Geometry check sheet. Reference: the model listing, model coordinates, mm. A direction names the side the tool comes from. Round coordinates to 2 decimals unless told otherwise and drop trailing zeros. Order: outer loops, then holes, each group sorted by start corner. A loop starts at its lowest first (then second) coordinate and runs counter-clockwise, first axis right, second up.
(1) Gauge pin test, flat ends, axial feed: P1, Ø3, axis at x = 28, y = -54, coming from the -Z side; P2, Ø8, axis at y = -20.5, z = 7.5, coming from the +X side; P3, Ø3, axis at y = -16.5, z = 34.5, coming from the +X side. Record the tip position at first contact, or that the pin passes through.
(2) Cross-section at C-C on x = 9.5. Enter the section's corners in (y, z).
(3) Cross-section at A-A on z = 12.7. Enter the section's corners in (x, y) (3 decimals), and give its area (3 significant figures).
(4) Cross-section at B-B on y = -12.7. Enter the section's corners in (x, z) (3 decimals), and give its area (3 significant figures).
(5) Thickness scan on L1, parallel to Z at x = 2.5, y = -76.2 (3 decimals); L2, parallel to Y at x = 5, z = 15.5; L3, parallel to Z at x = 36, y = -14. Record the ranges inside material, lowest first.
(6) Set-up check for faces 5 (the face through (11.81, -80.9, 35.67)), 6 (the face through (34, -44, 32.539)): record each of +Z, -Z, +X, -X, +Y, -Y from which the full face is reachable in a straight line by a thin tool's end or side.
(7) Cross-section at D-D on y = -56. Enter the section's corners in (x, z).
(8) Draft check along Z on faces 1 (the face through (13.465, -8.979, 35.669)), 2 (the face through (3.13, -86.32, 2.5)), 3 (the face through (3.13, -73.68, 10.77)), 4 (the face through (32, -44, 38.887)). Enter one of: pulls with the +Z half, pulls with the -Z half, needs draft (parallel to the pull), parting line crosses it, or undercut.
from build123d import *

# Parameters (mm, degrees)
F1_DEPTH = 88.9
F3_D     = 6.35
F4_SIZE  = 5.08
F6_D     = 6.35


with BuildPart() as f1:
    # F0 (on Front) → F1 (new body)
    with BuildSketch(Plane.XZ):
        Polygon((0, 38.8874), (0, 0), (6.35, 0), (6.35, 32.539288), (63.345166, 32.539288), (63.5, 38.8874), align=None)
    extrude(amount=F1_DEPTH)

    # F3 (through all)
    with Locations(Plane.YZ.offset(6.35)):
        with Locations((-76.2, 12.7), (-12.7, 12.7)):
            Hole(F3_D / 2)

    # F4
    f4_edges = [f1.edges().sort_by_distance(p)[0] for p in [
        (63.422583, 0, 35.713344),
        (63.422583, -88.9, 35.713344),
        (3.175, 0, 0),
        (3.175, -88.9, 0),
    ]]
    chamfer(f4_edges, length=F4_SIZE)

    # F6 (through all)
    with Locations(Plane.XY.offset(38.8874)):
        with Locations((11.1252, -11.1252), (25.4, -11.1252), (25.4, -77.8002), (11.1252, -77.8002)):
            Hole(F6_D / 2)


solid = f1.part
Found:
1. P1: stops at z = 32.54
1. P2: stops at x = 6.35
1. P3: stops at x = 63.43
2. outline: (-88.9, 32.54) - (-80.53, 32.54) - (-80.53, 38.89) - (-88.9, 38.89) - close; (-75.07, 32.54) - (-13.85, 32.54) - (-13.85, 38.89) - (-75.07, 38.89) - close; (-8.4, 32.54) - (0, 32.54) - (0, 38.89) - (-8.4, 38.89) - close
3. outline: (0, -88.9) - (6.35, -88.9) - (6.35, -79.375) - (0, -79.375) - close; (0, -73.025) - (6.35, -73.025) - (6.35, -15.875) - (0, -15.875) - close; (0, -9.525) - (6.35, -9.525) - (6.35, 0) - (0, 0) - close
3. area: 484 mm2
4. outline: (0, 0) - (6.35, 0) - (6.35, 9.525) - (0, 9.525) - close; (0, 15.875) - (6.35, 15.875) - (6.35, 32.539) - (8.368, 32.539) - (8.368, 38.887) - (0, 38.887) - close; (13.882, 32.539) - (22.643, 32.539) - (22.643, 38.887) - (13.882, 38.887) - close; (28.157, 32.539) - (63.345, 32.539) - (63.5, 38.887) - (28.157, 38.887) - close
4. area: 499 mm2
5. L1: z = 0 to 9.525, 15.875 to 38.887
5. L2: y = -88.9 to -77.7, -74.7 to -14.2, -11.2 to 0
5. L3: z = 32.54 to 38.89
6. face 5: +Z, -Z
6. face 6: -Z, +X, +Y, -Y
7. outline: (0, 0) - (6.35, 0) - (6.35, 32.54) - (63.35, 32.54) - (63.5, 38.89) - (0, 38.89) - close
8. face 1: needs draft
8. face 2: pulls with the -Z half
8. face 3: undercut
8. face 4: pulls with the +Z half
